Verification items for the finished model (mm, model axes). A direction names the side the tool comes from. Round coordinates to 2 decimals unless told otherwise and drop trailing zeros. Loops run counter-clockwise (first coordinate to the right, second up) from the corner with the lowest first, then second, coordinate; pieces in that order, holes last. Notation, with made-up numbers: (69.25, 19.25) -> (75.25, 19.25) arc R21 ccw to (75.25, 41.25) -> close; hole circle Ø5 at (58.25, -14). An arc over 180 degrees is marked (long way). Use a Markdown table: item, result. Add a question column.
```python
from build123d import *

# Parameters (mm, degrees)
EXTRUDE_1_DEPTH     = 13
SKETCH_2_R          = 31
CUT_EXTRUDE_3_DEPTH = 7
SKETCH_4_R          = 3
CUT_EXTRUDE_4_DEPTH = 31
CHAMFER_1_SIZE      = 10
CUT_EXTRUDE_5_DEPTH = 7
SKETCH_7_R          = 3
CUT_EXTRUDE_7_DEPTH = 80
FILLET_1_R          = 10
SKETCH_8_R          = 23.5
CUT_EXTRUDE_8_DEPTH = 10


with BuildPart() as part:
    # 草图1 → 拉伸1 (new body)
    with BuildSketch(Plane.XY):
        with BuildLine():
            Line((0, 55), (90, 55))
            ThreePointArc((90, 55), (145, 0), (90, -55))
            Line((90, -55), (0, -55))
            ThreePointArc((0, -55), (-55, 0), (0, 55))
        make_face()
    extrude(amount=EXTRUDE_1_DEPTH)

    # 草图2 → 切除-拉伸3 (cut)
    with BuildSketch(Plane.XY.offset(13)):
        with Locations((90, 0)):
            Circle(SKETCH_2_R)
    extrude(amount=-CUT_EXTRUDE_3_DEPTH, mode=Mode.SUBTRACT)

    # 草图4 → 切除-拉伸4 (cut)
    with BuildSketch(Plane(origin=(0, 0, 0), x_dir=(-1, 0, 0), z_dir=(0, 0, -1))):
        with Locations((-90, 22.5)):
            Circle(SKETCH_4_R)
        with Locations((-74.090097423, 15.909902577)):
            Circle(SKETCH_4_R)
        with Locations((-67.5, 0)):
            Circle(SKETCH_4_R)
        with Locations((-74.090097423, -15.909902577)):
            Circle(SKETCH_4_R)
        with Locations((-90, -22.5)):
            Circle(SKETCH_4_R)
        with Locations((-105.909902577, -15.909902577)):
            Circle(SKETCH_4_R)
        with Locations((-112.5, 0)):
            Circle(SKETCH_4_R)
        with Locations((-105.909902577, 15.909902577)):
            Circle(SKETCH_4_R)
    extrude(amount=-CUT_EXTRUDE_4_DEPTH, mode=Mode.SUBTRACT)

    # 倒角1
    chamfer_1_edges = [part.edges().sort_by_distance(p)[0] for p in [
        (45, 55, 0),
        (145, 0, 0),
        (45, -55, 0),
        (-55, 0, 0),
    ]]
    chamfer(chamfer_1_edges, length=CHAMFER_1_SIZE)

    # 草图5 → 切除-拉伸5 (cut)
    with BuildSketch(Plane.XY.offset(13)):
        with BuildLine():
            Line((50, 31), (90, 31))
            ThreePointArc((90, 31), (121, 0), (90, -31))
            Line((90, -31), (50, -31))
            Line((50, -31), (50, 31))
        make_face()
    extrude(amount=-CUT_EXTRUDE_5_DEPTH, mode=Mode.SUBTRACT)

    # 草图7 → 切除-拉伸7 (cut)
    with BuildSketch(Plane(origin=(0, 0, 0), x_dir=(-1, 0, 0), z_dir=(0, 0, -1))):
        with Locations((19.445436483, 19.445436483)):
            Circle(SKETCH_7_R)
        with Locations((27.5, 0)):
            Circle(SKETCH_7_R)
        with Locations((19.445436483, -19.445436483)):
            Circle(SKETCH_7_R)
        with Locations((0, -27.5)):
            Circle(SKETCH_7_R)
        with Locations((0, 27.5)):
            Circle(SKETCH_7_R)
        with Locations((-19.445436483, -19.445436483)):
            Circle(SKETCH_7_R)
        with Locations((-27.5, 0)):
            Circle(SKETCH_7_R)
        with Locations((-19.445436483, 19.445436483)):
            Circle(SKETCH_7_R)
    extrude(amount=-CUT_EXTRUDE_7_DEPTH, mode=Mode.SUBTRACT)

    # 圆角1
    fillet_1_edges = [part.edges().sort_by_distance(p)[0] for p in [
        (50, -31, 9.5),
        (50, 31, 9.5),
    ]]
    fillet(fillet_1_edges, radius=FILLET_1_R)

    # 草图8 → 切除-拉伸8 (cut)
    with BuildSketch(Plane.XY.offset(13)):
        Circle(SKETCH_8_R)
    extrude(amount=-CUT_EXTRUDE_8_DEPTH, mode=Mode.SUBTRACT)


solid = part.part
```
1) Go/stop test with flat-tipped pins: pin 1 (3.5 mm diameter, centred on x = -27.5, y = 0, fed in from -Z); pin 2 (8 mm diameter, centred on x = 105.91, y = 15.91, fed in from -Z); pin 3 (2 mm diameter, centred on y = -4.5, z = 9.5, fed in from +X); pin 4 (6 mm diameter, centred on y = -6, z = 1.5, fed in from +X). Record where each tip stops, or that it passes through.
2) Sectioned sample at B-B on x = -19. State how many separate pieces and enclosed holes the cut face has, then the cut area to 3 significant figures.
3) Release check for a two-part mould opening along X. For faces 1 (the face through (-54.987, -1.209, 11.479)), 2 (the face through (52.85, 27.99, 9.45)), 3 (the face through (144.987, 1.209, 11.479)), 4 (the face through (120.993, -0.682, 9.549)) record: released by +X, released by -X, zero draft, split by the parting line, or undercut.
4) Sectioned sample at A-A on x = 27.5. Enter the section's corners in (y, z).
5) Access from +Z, -Z, +X, -X, +Y, -Y to the whole of each face (thin tool, end or side, straight path). Record for faces 5 (the face through (16.674, -20.594, 6.409)), 6 (the face through (0, 0, 3)).
6) Thickness scan on line 1 (Y direction, x = -2, z = 3.5); line 2 (Y direction, x = 0, z = 9.5); line 3 (Y direction, x = 84.5, z = 10). Record the ranges inside material, lowest first.
Geometry results:
| question | item | result |
|---|---|---|
| 1 | pin 1 | through |
| 1 | pin 2 | z = 0 |
| 1 | pin 3 | x = 144.88 |
| 1 | pin 4 | x = 139.16 |
| 2 | separate pieces | 3 |
| 2 | enclosed holes | 0 |
| 2 | area | 804 mm^2 |
| 3 | face 1 | released by -X |
| 3 | face 2 | undercut |
| 3 | face 3 | released by +X |
| 3 | face 4 | undercut |
| 4 | outline | (-55, 10) -> (-45, 0) -> (-3, 0) -> (-3, 13) -> (-55, 13) -> close; (3, 0) -> (45, 0) -> (55, 10) -> (55, 13) -> (3, 13) -> close |
| 5 | face 5 | +Z, -Z |
| 5 | face 6 | +Z |
| 6 | line 1 | -48.46 to -29.74, -25.26 to -23.41, 23.41 to 25.26, 29.74 to 48.46 |
| 6 | line 2 | -54.5 to -30.5, -24.5 to -23.5, 23.5 to 24.5, 30.5 to 54.5 |
| 6 | line 3 | -55 to -31, 31 to 55 |
